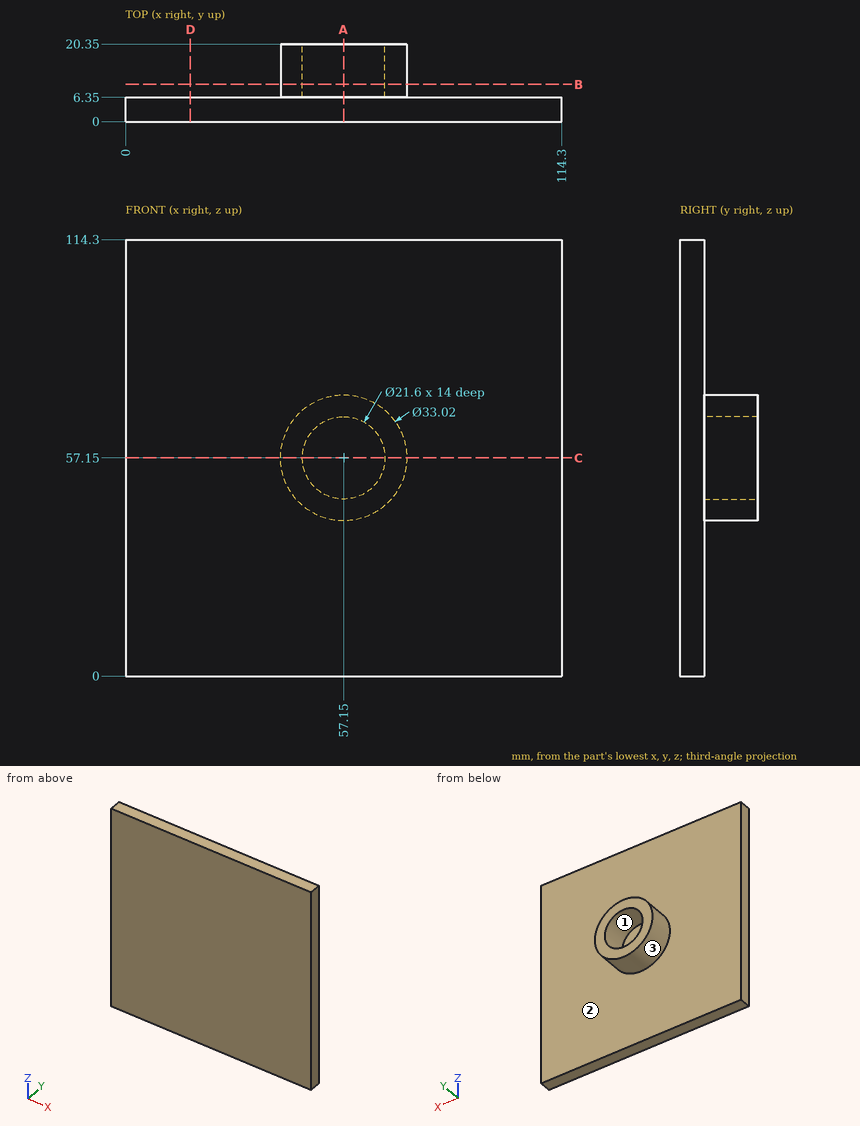
Could you check a few things on this drawing? It's one solid part, dimensions in mm from its lowest x, y, z. Coordinates: 2 decimals unless noted, no trailing zeros. Loops run counter-clockwise (first coordinate to the right, second up) from the corner with the lowest first, then second, coordinate; pieces in that order, holes last. Notation, with made-up numbers: (-37, 36) - (-6, 36) arc R8 cw to (-6, 43) - close; hole circle Ø10 at (72.25, -17). An arc over 180 degrees is marked (long way). Answer as a JSON object with one key per item and string values. Group by question number.
Item 1: If we section it at B-B (y = 9.75): List the corners of the cut face in (x, z) for me, plus the area to 3 significant figures.
Item 2: For pin 1 (6 mm diameter, centred on x = 25, z = 34, fed in from +Y); pin 2 (10 mm diameter, centred on y = 13, z = 23, fed in from -X); pin 3 (19.5 mm diameter, centred on x = 57.15, z = 57.15, fed in from +Y); pin 4 (3 mm diameter, centred on x = 65.5, y = 8.5, fed in from -Z), each with a flat end and sliding along its axis, tell me the tip position at first contact or that it passes through.
Item 3: If we section it at A-A (x = 57.15): List the corners of the cut face in (y, z) for me.
Item 4: If I drill on L1, parallel to X at y = 10.25, z = 57.15; L2, parallel to Y at x = 51, z = 106.5; L3, parallel to X at y = 12.5, z = 62, over which ranges is the centre line in solid material (lowest first)? Write a range as from..to.
Item 5: If we section it at D-D (x = 17): List the corners of the cut face in (y, z) for me.
Item 6: If we section it at C-C (z = 57.15): List the corners of the cut face in (x, y) for me.
Item 7: If we mould it in two halves opening along Z, with no side actions, what happens to the marked faces 1, 2 and 3? For each: released by +Z, released by -Z, zero draft, split by the parting line, or undercut.
Returned:
{
 "1": {"outline": "circle Ø33.02 at (57.15, 57.15); hole circle Ø21.6 at (57.15, 57.15)", "area": "490 mm²"},
 "2": {"pin 1": "stops at y = 6.35", "pin 2": "passes through", "pin 3": "stops at y = 6.35", "pin 4": "stops at z = 42.13"},
 "3": {"outline": "(0, 0) - (6.35, 0) - (6.35, 40.64) - (20.35, 40.64) - (20.35, 46.35) - (6.35, 46.35) - (6.35, 67.95) - (20.35, 67.95) - (20.35, 73.66) - (6.35, 73.66) - (6.35, 114.3) - (0, 114.3) - close"},
 "4": {"L1": "x = 40.64..46.35, 67.95..73.66", "L2": "y = 0..6.35", "L3": "x = 41.37..47.5, 66.8..72.93"},
 "5": {"outline": "(0, 0) - (6.35, 0) - (6.35, 114.3) - (0, 114.3) - close"},
 "6": {"outline": "(0, 0) - (114.3, 0) - (114.3, 6.35) - (73.66, 6.35) - (73.66, 20.35) - (67.95, 20.35) - (67.95, 6.35) - (46.35, 6.35) - (46.35, 20.35) - (40.64, 20.35) - (40.64, 6.35) - (0, 6.35) - close"},
 "7": {"face 1": "undercut", "face 2": "zero draft", "face 3": "split by the parting line"}
}
